```python
from build123d import *

# Parameters (mm, degrees)
CHAFL_N1_SIZE         = 2
CORTAR_EXTRUIR1_REACH = 190.482


with BuildPart() as part:
    # Croquis1 → Revolución1 (revolve)
    with BuildSketch(Plane.XY, mode=Mode.PRIVATE) as revoluci_n1_sk:
        Polygon((0, 0), (188, 0), (188, 6), (5, 6), (5, 9.525), (0, 9.525), align=None)
    revolve(revoluci_n1_sk.sketch.rotate(Axis((0, 0, 0), (1, 0, 0)), 90), axis=Axis((0, 0, 0), (1, 0, 0)))

    # Chaflán1
    chafl_n1_edges = [part.edges().sort_by_distance(p)[0] for p in [
        (188, 0, -6),
    ]]
    chamfer(chafl_n1_edges, length=CHAFL_N1_SIZE)

    # Croquis2 → Cortar-Extruir1 (cut, up to next)
    with BuildSketch(Plane.ZY, mode=Mode.PRIVATE) as cortar_extruir1_sk1:
        with BuildLine():
            Line((-4.298328163, 8.5), (4.298328163, 8.5))
            ThreePointArc((4.298328163, 8.5), (0, 9.525), (-4.298328163, 8.5))
        make_face()
    cortar_extruir1_tool1 = extrude(cortar_extruir1_sk1.sketch, amount=-CORTAR_EXTRUIR1_REACH, mode=Mode.PRIVATE) & part.part
    # Croquis2 → Cortar-Extruir1 (cut, up to next)
    with BuildSketch(Plane.ZY, mode=Mode.PRIVATE) as cortar_extruir1_sk2:
        with BuildLine():
            Line((-9.510380014, 0.527538617), (-5.21205185, 7.972461383))
            ThreePointArc((-5.21205185, 7.972461383), (-8.248891971, 4.7625), (-9.510380014, 0.527538617))
        make_face()
    cortar_extruir1_tool2 = extrude(cortar_extruir1_sk2.sketch, amount=-CORTAR_EXTRUIR1_REACH, mode=Mode.PRIVATE) & part.part
    # Croquis2 → Cortar-Extruir1 (cut, up to next)
    with BuildSketch(Plane.ZY, mode=Mode.PRIVATE) as cortar_extruir1_sk3:
        with BuildLine():
            Line((-5.21205185, -7.972461383), (-9.510380014, -0.527538617))
            ThreePointArc((-9.510380014, -0.527538617), (-8.248891971, -4.7625), (-5.21205185, -7.972461383))
        make_face()
    cortar_extruir1_tool3 = extrude(cortar_extruir1_sk3.sketch, amount=-CORTAR_EXTRUIR1_REACH, mode=Mode.PRIVATE) & part.part
    # Croquis2 → Cortar-Extruir1 (cut, up to next)
    with BuildSketch(Plane.ZY, mode=Mode.PRIVATE) as cortar_extruir1_sk4:
        with BuildLine():
            ThreePointArc((-4.298328163, -8.5), (0, -9.525), (4.298328163, -8.5))
            Line((4.298328163, -8.5), (-4.298328163, -8.5))
        make_face()
    cortar_extruir1_tool4 = extrude(cortar_extruir1_sk4.sketch, amount=-CORTAR_EXTRUIR1_REACH, mode=Mode.PRIVATE) & part.part
    # Croquis2 → Cortar-Extruir1 (cut, up to next)
    with BuildSketch(Plane.ZY, mode=Mode.PRIVATE) as cortar_extruir1_sk5:
        with BuildLine():
            ThreePointArc((5.21205185, -7.972461383), (8.248891971, -4.7625), (9.510380014, -0.527538617))
            Line((9.510380014, -0.527538617), (5.21205185, -7.972461383))
        make_face()
    cortar_extruir1_tool5 = extrude(cortar_extruir1_sk5.sketch, amount=-CORTAR_EXTRUIR1_REACH, mode=Mode.PRIVATE) & part.part
    # Croquis2 → Cortar-Extruir1 (cut, up to next)
    with BuildSketch(Plane.ZY, mode=Mode.PRIVATE) as cortar_extruir1_sk6:
        with BuildLine():
            ThreePointArc((9.510380014, 0.527538617), (8.248891971, 4.7625), (5.21205185, 7.972461383))
            Line((5.21205185, 7.972461383), (9.510380014, 0.527538617))
        make_face()
    cortar_extruir1_tool6 = extrude(cortar_extruir1_sk6.sketch, amount=-CORTAR_EXTRUIR1_REACH, mode=Mode.PRIVATE) & part.part
    add(cortar_extruir1_tool1.solids().sort_by_distance((0, 8.911952, 0))[0], mode=Mode.SUBTRACT)
    add(cortar_extruir1_tool2.solids().sort_by_distance((0, 4.455976, -7.717977))[0], mode=Mode.SUBTRACT)
    add(cortar_extruir1_tool3.solids().sort_by_distance((0, -4.455976, -7.717977))[0], mode=Mode.SUBTRACT)
    add(cortar_extruir1_tool4.solids().sort_by_distance((0, -8.911952, 0))[0], mode=Mode.SUBTRACT)
    add(cortar_extruir1_tool5.solids().sort_by_distance((0, -4.455976, 7.717977))[0], mode=Mode.SUBTRACT)
    add(cortar_extruir1_tool6.solids().sort_by_distance((0, 4.455976, 7.717977))[0], mode=Mode.SUBTRACT)


solid = part.part
```
Design review of the part built by this model. Coordinates are the model's own, in mm. A direction names the side the tool comes from. Give positions to 0.01 mm unless a question says otherwise; leave off trailing zeros. Order: outer loops, then holes, each group sorted by start corner. A loop starts at its lowest first (then second) coordinate and runs counter-clockwise, first axis right, second up. Notation, with made-up numbers: (72.25, 60.25) - (116.25, 60.25) arc R17 cw to (116.25, 66.25) - close; hole circle Ø1 at (46, -29.75). An arc over 180 degrees is marked (long way). Use a Markdown table: item, result. Add a question column.
(1) Add section A-A on z = 0. Give the boundary of the cut face in (x, y), then the cut area to 3 significant figures.
(2) Clearance check with flat-ended pins moving along their axes: P1, Ø6, axis at x = 80, z = 2, coming from the -Y side; P2, Ø5, axis at x = 47.5, y = -2.5, coming from the +Z side; P3, Ø3, axis at x = 81, z = 2.5, coming from the -Y side. State where each tip first meets the part, or that it passes through.
(3) Machinability: for faces 1 (the face through (94.233, -1.802, 5.723)), 2 (the face through (0, 0, 0)), which of the approach directions +Z, -Z, +X, -X, +Y, -Y give a long, thin tool a straight path to every point of the face, cutting with its end or side? Answer none if there is none.
(4) Wall thickness on probe 1 along X at (y, z) = (2.25, 6.75); probe 2 along Y at (x, z) = (68.5, -4.5); probe 3 along Z at (x, y) = (156.5, 0.25): over which ranges is each line inside the solid? List them lowest first. Write a range as [from, to].
(5) Add section B-B on x = 145.5. Give the boundary of the cut face in (y, z).
Report:
| question | item | result |
|---|---|---|
| 1 | outline | (0, -8.5) - (5, -8.5) - (5, -6) - (186, -6) - (188, -4) - (188, 4) - (186, 6) - (5, 6) - (5, 8.5) - (0, 8.5) - close |
| 1 | area | 2,280 mm² |
| 2 | P1 | stops at y = -6 |
| 2 | P2 | stops at z = 6 |
| 2 | P3 | stops at y = -5.92 |
| 3 | face 1 | +X |
| 3 | face 2 | +Z, -Z, -X, +Y, -Y |
| 4 | probe 1 | x = [0, 5] |
| 4 | probe 2 | y = [-3.97, 3.97] |
| 4 | probe 3 | z = [-5.99, 5.99] |
| 5 | outline | circle Ø12 at (0, 0) |
